from build123d import *

# Parameters (mm, degrees)
CYLINDER025_R             = 0.5
CYLINDER025_DEPTH         = 10
CYLINDER026_R             = 0.5
CYLINDER026_DEPTH         = 10
CYLINDER027_R             = 0.5
CYLINDER027_DEPTH         = 10
CYLINDER024_R             = 0.5
CYLINDER024_DEPTH         = 10
CYLINDER007_R             = 1.5
CYLINDER007_DEPTH         = 10
CYLINDER008_R             = 1.5
CYLINDER008_DEPTH         = 10
CYLINDER009_R             = 1.5
CYLINDER009_DEPTH         = 10
CYLINDER006_R             = 1.5
CYLINDER006_DEPTH         = 10
BOX002_W                  = 3
BOX002_H                  = 6
BOX002_DEPTH              = 10
CYLINDER010_R             = 1.5
CYLINDER010_DEPTH         = 10
CYLINDER011_R             = 1.5
CYLINDER011_DEPTH         = 10
CYLINDER005_R             = 1.5
CYLINDER005_DEPTH         = 10
BOX001_W                  = 6
BOX001_H                  = 3
BOX001_DEPTH              = 10
CYLINDER004_R             = 1.5
CYLINDER004_DEPTH         = 10
BOX005_W                  = 29
BOX005_H                  = 31
BOX005_DEPTH              = 3
CYLINDER021_R             = 0.5
CYLINDER021_DEPTH         = 10
CYLINDER022_R             = 0.5
CYLINDER022_DEPTH         = 10
CYLINDER023_R             = 0.5
CYLINDER023_DEPTH         = 10
CYLINDER020_R             = 0.5
CYLINDER020_DEPTH         = 10
CYLINDER016_R             = 1.5
CYLINDER016_DEPTH         = 10
CYLINDER015_R             = 1.5
CYLINDER015_DEPTH         = 10
CYLINDER018_R             = 1.5
CYLINDER018_DEPTH         = 10
CYLINDER014_R             = 1.5
CYLINDER014_DEPTH         = 10
BOX004_W                  = 3
BOX004_H                  = 6
BOX004_DEPTH              = 10
CYLINDER017_R             = 1.5
CYLINDER017_DEPTH         = 10
CYLINDER019_R             = 1.5
CYLINDER019_DEPTH         = 10
CYLINDER012_R             = 1.5
CYLINDER012_DEPTH         = 10
BOX003_W                  = 6
BOX003_H                  = 3
BOX003_DEPTH              = 10
CYLINDER013_R             = 1.5
CYLINDER013_DEPTH         = 10
FUSION008_PLACEMENT_ANGLE = 180
BOX006_W                  = 25
BOX006_H                  = 31
BOX006_DEPTH              = 3
CYLINDER003_R             = 0.75
CYLINDER003_DEPTH         = 10
CYLINDER002_R             = 0.75
CYLINDER002_DEPTH         = 10
CYLINDER001_R             = 1.3
CYLINDER001_DEPTH         = 10
CYLINDER_R                = 2.5
CYLINDER_DEPTH            = 10
BOX_W                     = 27
BOX_H                     = 31
BOX_DEPTH                 = 2
CHAMFER_SIZE              = 5
CHAMFER001_SIZE           = 5
CHAMFER002_SIZE           = 0.99


with BuildPart() as zylinder025:
    # Cylinder025 → Cylinder025 (new body)
    with BuildSketch(Plane(origin=(-41, -22.5, 0), x_dir=(1, 0, 0), z_dir=(0, 0, 1))):
        Circle(CYLINDER025_R)
    extrude(amount=CYLINDER025_DEPTH)


with BuildPart() as zylinder026:
    # Cylinder026 → Cylinder026 (new body)
    with BuildSketch(Plane(origin=(-28, -12, 0), x_dir=(1, 0, 0), z_dir=(0, 0, 1))):
        Circle(CYLINDER026_R)
    extrude(amount=CYLINDER026_DEPTH)


with BuildPart() as zylinder027:
    # Cylinder027 → Cylinder027 (new body)
    with BuildSketch(Plane(origin=(-28, -22.5, 0), x_dir=(1, 0, 0), z_dir=(0, 0, 1))):
        Circle(CYLINDER027_R)
    extrude(amount=CYLINDER027_DEPTH)


with BuildPart() as fusion010:
    # Cylinder024 → Cylinder024 (new body)
    with BuildSketch(Plane(origin=(-41, -12, 0), x_dir=(1, 0, 0), z_dir=(0, 0, 1))):
        Circle(CYLINDER024_R)
    extrude(amount=CYLINDER024_DEPTH)

    # Fusion010: union Zylinder025, Zylinder026, Zylinder027
    add(zylinder025.part)
    add(zylinder026.part)
    add(zylinder027.part)


with BuildPart() as fusion010_1:
    # Fusion010 placement: moved
    add(fusion010.part.moved(Location((50, -0.5, 0))))


with BuildPart() as zylinder007:
    # Cylinder007 → Cylinder007 (new body)
    with BuildSketch(Plane(origin=(18.7, -24, 0), x_dir=(1, 0, 0), z_dir=(0, 0, 1))):
        Circle(CYLINDER007_R)
    extrude(amount=CYLINDER007_DEPTH)


with BuildPart() as zylinder008:
    # Cylinder008 → Cylinder008 (new body)
    with BuildSketch(Plane(origin=(18.7, -28.5, 0), x_dir=(1, 0, 0), z_dir=(0, 0, 1))):
        Circle(CYLINDER008_R)
    extrude(amount=CYLINDER008_DEPTH)


with BuildPart() as zylinder009:
    # Cylinder009 → Cylinder009 (new body)
    with BuildSketch(Plane(origin=(11.7, -28.5, 0), x_dir=(1, 0, 0), z_dir=(0, 0, 1))):
        Circle(CYLINDER009_R)
    extrude(amount=CYLINDER009_DEPTH)


with BuildPart() as fusion002:
    # Cylinder006 → Cylinder006 (new body)
    with BuildSketch(Plane(origin=(11.7, -24, 0), x_dir=(1, 0, 0), z_dir=(0, 0, 1))):
        Circle(CYLINDER006_R)
    extrude(amount=CYLINDER006_DEPTH)

    # Fusion002: union Zylinder007, Zylinder008, Zylinder009
    add(zylinder007.part)
    add(zylinder008.part)
    add(zylinder009.part)


with BuildPart() as obj1:
    # Box002 → Box002 (new body)
    with BuildSketch(Plane(origin=(23, -20.5, 0), x_dir=(1, 0, 0), z_dir=(0, 0, 1))):
        with Locations((1.5, 3)):
            Rectangle(BOX002_W, BOX002_H)
    extrude(amount=BOX002_DEPTH)


with BuildPart() as zylinder010:
    # Cylinder010 → Cylinder010 (new body)
    with BuildSketch(Plane(origin=(24.5, -14.5, 0), x_dir=(1, 0, 0), z_dir=(0, 0, 1))):
        Circle(CYLINDER010_R)
    extrude(amount=CYLINDER010_DEPTH)


with BuildPart() as fusion003:
    # Cylinder011 → Cylinder011 (new body)
    with BuildSketch(Plane(origin=(24.5, -20.5, 0), x_dir=(1, 0, 0), z_dir=(0, 0, 1))):
        Circle(CYLINDER011_R)
    extrude(amount=CYLINDER011_DEPTH)

    # Fusion003: union obj1, Zylinder010
    add(obj1.part)
    add(zylinder010.part)


with BuildPart() as zylinder005:
    # Cylinder005 → Cylinder005 (new body)
    with BuildSketch(Plane(origin=(18, -8.7, 0), x_dir=(1, 0, 0), z_dir=(0, 0, 1))):
        Circle(CYLINDER005_R)
    extrude(amount=CYLINDER005_DEPTH)


with BuildPart() as obj2:
    # Box001 → Box001 (new body)
    with BuildSketch(Plane(origin=(12, -10.2, 0), x_dir=(1, 0, 0), z_dir=(0, 0, 1))):
        with Locations((3, 1.5)):
            Rectangle(BOX001_W, BOX001_H)
    extrude(amount=BOX001_DEPTH)


with BuildPart() as fusion011:
    # Cylinder004 → Cylinder004 (new body)
    with BuildSketch(Plane(origin=(12, -8.7, 0), x_dir=(1, 0, 0), z_dir=(0, 0, 1))):
        Circle(CYLINDER004_R)
    extrude(amount=CYLINDER004_DEPTH)

    # Fusion001: union Zylinder005, obj2
    add(zylinder005.part)
    add(obj2.part)

    # Fusion004: union Fusion002, Fusion003
    add(fusion002.part)
    add(fusion003.part)

    # Fusion011: union Fusion010
    add(fusion010_1.part)


with BuildPart() as cut003:
    # Box005 → Box005 (new body)
    with BuildSketch(Plane(origin=(1, -33, 0), x_dir=(1, 0, 0), z_dir=(0, 0, 1))):
        with Locations((14.5, 15.5)):
            Rectangle(BOX005_W, BOX005_H)
    extrude(amount=BOX005_DEPTH)

    # Cut003: cut Fusion011
    add(fusion011.part, mode=Mode.SUBTRACT)


with BuildPart() as zylinder021:
    # Cylinder021 → Cylinder021 (new body)
    with BuildSketch(Plane(origin=(-41, -22.5, 0), x_dir=(1, 0, 0), z_dir=(0, 0, 1))):
        Circle(CYLINDER021_R)
    extrude(amount=CYLINDER021_DEPTH)


with BuildPart() as zylinder022:
    # Cylinder022 → Cylinder022 (new body)
    with BuildSketch(Plane(origin=(-28, -12, 0), x_dir=(1, 0, 0), z_dir=(0, 0, 1))):
        Circle(CYLINDER022_R)
    extrude(amount=CYLINDER022_DEPTH)


with BuildPart() as zylinder023:
    # Cylinder023 → Cylinder023 (new body)
    with BuildSketch(Plane(origin=(-28, -22.5, 0), x_dir=(1, 0, 0), z_dir=(0, 0, 1))):
        Circle(CYLINDER023_R)
    extrude(amount=CYLINDER023_DEPTH)


with BuildPart() as fusion009:
    # Cylinder020 → Cylinder020 (new body)
    with BuildSketch(Plane(origin=(-41, -12, 0), x_dir=(1, 0, 0), z_dir=(0, 0, 1))):
        Circle(CYLINDER020_R)
    extrude(amount=CYLINDER020_DEPTH)

    # Fusion009: union Zylinder021, Zylinder022, Zylinder023
    add(zylinder021.part)
    add(zylinder022.part)
    add(zylinder023.part)


with BuildPart() as zylinder016:
    # Cylinder016 → Cylinder016 (new body)
    with BuildSketch(Plane(origin=(18.7, -24, 0), x_dir=(1, 0, 0), z_dir=(0, 0, 1))):
        Circle(CYLINDER016_R)
    extrude(amount=CYLINDER016_DEPTH)


with BuildPart() as zylinder015:
    # Cylinder015 → Cylinder015 (new body)
    with BuildSketch(Plane(origin=(18.7, -28.5, 0), x_dir=(1, 0, 0), z_dir=(0, 0, 1))):
        Circle(CYLINDER015_R)
    extrude(amount=CYLINDER015_DEPTH)


with BuildPart() as zylinder018:
    # Cylinder018 → Cylinder018 (new body)
    with BuildSketch(Plane(origin=(11.7, -28.5, 0), x_dir=(1, 0, 0), z_dir=(0, 0, 1))):
        Circle(CYLINDER018_R)
    extrude(amount=CYLINDER018_DEPTH)


with BuildPart() as fusion006:
    # Cylinder014 → Cylinder014 (new body)
    with BuildSketch(Plane(origin=(11.7, -24, 0), x_dir=(1, 0, 0), z_dir=(0, 0, 1))):
        Circle(CYLINDER014_R)
    extrude(amount=CYLINDER014_DEPTH)

    # Fusion006: union Zylinder016, Zylinder015, Zylinder018
    add(zylinder016.part)
    add(zylinder015.part)
    add(zylinder018.part)


with BuildPart() as obj3:
    # Box004 → Box004 (new body)
    with BuildSketch(Plane(origin=(23, -20.5, 0), x_dir=(1, 0, 0), z_dir=(0, 0, 1))):
        with Locations((1.5, 3)):
            Rectangle(BOX004_W, BOX004_H)
    extrude(amount=BOX004_DEPTH)


with BuildPart() as zylinder017:
    # Cylinder017 → Cylinder017 (new body)
    with BuildSketch(Plane(origin=(24.5, -14.5, 0), x_dir=(1, 0, 0), z_dir=(0, 0, 1))):
        Circle(CYLINDER017_R)
    extrude(amount=CYLINDER017_DEPTH)


with BuildPart() as fusion007:
    # Cylinder019 → Cylinder019 (new body)
    with BuildSketch(Plane(origin=(24.5, -20.5, 0), x_dir=(1, 0, 0), z_dir=(0, 0, 1))):
        Circle(CYLINDER019_R)
    extrude(amount=CYLINDER019_DEPTH)

    # Fusion007: union obj3, Zylinder017
    add(obj3.part)
    add(zylinder017.part)


with BuildPart() as zylinder012:
    # Cylinder012 → Cylinder012 (new body)
    with BuildSketch(Plane(origin=(18, -8.7, 0), x_dir=(1, 0, 0), z_dir=(0, 0, 1))):
        Circle(CYLINDER012_R)
    extrude(amount=CYLINDER012_DEPTH)


with BuildPart() as obj4:
    # Box003 → Box003 (new body)
    with BuildSketch(Plane(origin=(12, -10.2, 0), x_dir=(1, 0, 0), z_dir=(0, 0, 1))):
        with Locations((3, 1.5)):
            Rectangle(BOX003_W, BOX003_H)
    extrude(amount=BOX003_DEPTH)


with BuildPart() as fusion012:
    # Cylinder013 → Cylinder013 (new body)
    with BuildSketch(Plane(origin=(12, -8.7, 0), x_dir=(1, 0, 0), z_dir=(0, 0, 1))):
        Circle(CYLINDER013_R)
    extrude(amount=CYLINDER013_DEPTH)

    # Fusion005: union Zylinder012, obj4
    add(zylinder012.part)
    add(obj4.part)

    # Fusion008: union Fusion006, Fusion007
    add(fusion006.part)
    add(fusion007.part)


with BuildPart() as fusion012_1:
    # Fusion008 placement: moved
    add(fusion012.part.moved(Location((-19, -35, 0))).rotate(Axis((-19, -35, 0), (0, 0, 1)), FUSION008_PLACEMENT_ANGLE))

    # Fusion012: union Fusion009
    add(fusion009.part)


with BuildPart() as cut004:
    # Box006 → Box006 (new body)
    with BuildSketch(Plane(origin=(-49, -33, 0), x_dir=(1, 0, 0), z_dir=(0, 0, 1))):
        with Locations((12.5, 15.5)):
            Rectangle(BOX006_W, BOX006_H)
    extrude(amount=BOX006_DEPTH)

    # Cut004: cut Fusion012
    add(fusion012_1.part, mode=Mode.SUBTRACT)


with BuildPart() as zylinder003:
    # Cylinder003 → Cylinder003 (new body)
    with BuildSketch(Plane(origin=(-14.7, -30, 0), x_dir=(1, 0, 0), z_dir=(0, 0, 1))):
        Circle(CYLINDER003_R)
    extrude(amount=CYLINDER003_DEPTH)


with BuildPart() as fusion:
    # Cylinder002 → Cylinder002 (new body)
    with BuildSketch(Plane(origin=(-2.7, -30, 0), x_dir=(1, 0, 0), z_dir=(0, 0, 1))):
        Circle(CYLINDER002_R)
    extrude(amount=CYLINDER002_DEPTH)

    # Fusion: union Zylinder003
    add(zylinder003.part)


with BuildPart() as zylinder001:
    # Cylinder001 → Cylinder001 (new body)
    with BuildSketch(Plane(origin=(-9.6, -15.8, 0), x_dir=(1, 0, 0), z_dir=(0, 0, 1))):
        Circle(CYLINDER001_R)
    extrude(amount=CYLINDER001_DEPTH)


with BuildPart() as zylinder:
    # Cylinder → Cylinder (new body)
    with BuildSketch(Plane(origin=(-16.4, -19.4, 0), x_dir=(1, 0, 0), z_dir=(0, 0, 1))):
        Circle(CYLINDER_R)
    extrude(amount=CYLINDER_DEPTH)


with BuildPart() as plate:
    # Box → Box (new body)
    with BuildSketch(Plane(origin=(-25, -33, 1), x_dir=(1, 0, 0), z_dir=(0, 0, 1))):
        with Locations((13.5, 15.5)):
            Rectangle(BOX_W, BOX_H)
    extrude(amount=BOX_DEPTH)

    # Cut: cut Zylinder
    add(zylinder.part, mode=Mode.SUBTRACT)

    # Cut001: cut Zylinder001
    add(zylinder001.part, mode=Mode.SUBTRACT)

    # Cut002: cut Fusion
    add(fusion.part, mode=Mode.SUBTRACT)

    # Fusion013: union Cut003, Cut004
    add(cut003.part)
    add(cut004.part)

    # Chamfer
    chamfer_edges = [plate.edges().sort_by_distance(p)[0] for p in [
        (30, -33, 1.5),
        (30, -2, 1.5),
    ]]
    chamfer(chamfer_edges, length=CHAMFER_SIZE)

    # Chamfer001
    chamfer001_edges = [plate.edges().sort_by_distance(p)[0] for p in [
        (-49, -33, 1.5),
        (-49, -2, 1.5),
    ]]
    chamfer(chamfer001_edges, length=CHAMFER001_SIZE)

    # Chamfer002
    chamfer002_edges = [plate.edges().sort_by_distance(p)[0] for p in [
        (-24, -17.5, 0),
        (1, -17.5, 0),
    ]]
    chamfer(chamfer002_edges, length=CHAMFER002_SIZE)


solid = plate.part
Design review of the part built by this model. Coordinates are the model's own, in mm. A direction names the side the tool comes from. Round coordinates to 2 decimals unless told otherwise and drop trailing zeros. Loops run counter-clockwise (first coordinate to the right, second up) from the corner with the lowest first, then second, coordinate; pieces in that order, holes last. Notation, with made-up numbers: (-30, 5) - (5, 5) arc R31 cw to (5, 39) - close; hole circle Ø10 at (72, 49.5). An arc over 180 degrees is marked (long way). One line per item, written item: value. Start each with the question number.
1) Insertion check: pin 1 Ø12.5 at (x, y) = (-9.5, -14) entering from -Z. The pin has a flat end and moves straight along its axis. Give the tip position at first contact, or say it passes through.
2) Consider section A-A on x = 14. Give the boundary of the cut face in (y, z).
3) Consider section B-B on y = -19.4. Give the number of separate pieces and of enclosed holes in the cut face, then the cut area to 3 significant figures.
4) Draft analysis for pull direction Y (two halves, no side actions). For faces 1 (the flat face through (-12, -17, 1)), 2 (the cylindrical face through (11.505, -27.013, 1.479)), 3 (the flat face through (27, -31, 1)), state which applies: +Y half, -Y half, draft (parallel to the pull), parting line (faces both ways), or undercut.
5) To check wall thickness, follow L1, parallel to Y at x = -41, z = 1.95; L2, parallel to Y at x = -30.7, z = 1.05; L3, parallel to X at y = -24.5, z = 2.05. State the ranges of each line that lie inside material, in increasing order. Write a range as from..to.
6) For faces 4 (the cylindrical face through (-38.5, -26.3, 1.5)), 5 (the flat face through (-10, -33, 1.5)), list the 3-axis set-ups (+Z, -Z, +X, -X, +Y, -Y) from which the entire face can be reached by the end or side of a thin tool; tool diameter is ignored.
7) Consider section D-D on x = -2.7. Give the boundary of the cut face in (y, z), then the cut area to 3 significant figures.
Reported:
1. pin 1: stops at z = 1
2. outline: (-33, 0) - (-10.2, 0) - (-10.2, 3) - (-33, 3) - close; (-7.2, 0) - (-2, 0) - (-2, 3) - (-7.2, 3) - close
3. separate pieces: 4
3. enclosed holes: 0
3. area: 183 mm^2
4. face 1: draft
4. face 2: undercut
4. face 3: -Y half
5. L1: y = -33..-23, -22..-12.5, -11.5..-2
5. L2: y = -33..-27.77, -24.83..-12.5, -9.5..-8, -5..-2
5. L3: x = -49..10.29, 13.11..17.29, 20.11..30
6. face 4: +Z, -Z
6. face 5: +Z, -Z, +X, -X, -Y
7. outline: (-33, 1) - (-30.75, 1) - (-30.75, 3) - (-33, 3) - close; (-29.25, 1) - (-2, 1) - (-2, 3) - (-29.25, 3) - close
7. area: 59.0 mm^2
